```python
from build123d import *

# Parameters (mm, degrees)
F0_W      = 12
F0_H      = 10
F1_DEPTH  = 3.3
F2_SIZE   = 2
F3_R      = 3
F4_R      = 3
F5_R      = 1.75
F6_DEPTH  = 25
F7_R      = 2.5
F8_DEPTH  = 25
F9_R      = 4.5
F10_DEPTH = 25
F10_TAPER = 10


with BuildPart() as f1:
    # F0 (on Top) → F1 (new body)
    with BuildSketch(Plane.XY):
        Polygon((15, -41), (15, 41), (3, 41), (-15, 41), (-15, -41), (-3, -41), align=None)
        with Locations((9, 46)):
            Rectangle(F0_W, F0_H)
        with Locations((-9, -46)):
            Rectangle(F0_W, F0_H)
    extrude(amount=F1_DEPTH)

    # F2
    f2_edges = [f1.edges().sort_by_distance(p)[0] for p in [
        (15, 51, 1.65),
        (3, 51, 1.65),
        (-15, -51, 1.65),
        (-3, -51, 1.65),
    ]]
    chamfer(f2_edges, length=F2_SIZE)

    # F3
    f3_edges = [f1.edges().sort_by_distance(p)[0] for p in [
        (3, 41, 1.65),
    ]]
    fillet(f3_edges, radius=F3_R)

    # F4
    f4_edges = [f1.edges().sort_by_distance(p)[0] for p in [
        (-3, -41, 1.65),
    ]]
    fillet(f4_edges, radius=F4_R)

    # F5 (on face) → F6 (cut)
    with BuildSketch(Plane.XY.offset(3.3)):
        with Locations((9, 46)):
            Circle(F5_R)
        with Locations((-9, -46)):
            Circle(F5_R)
    extrude(amount=-F6_DEPTH, mode=Mode.SUBTRACT)

    # F7 (on face) → F8 (cut)
    with BuildSketch(Plane.XY.offset(3.3)):
        with Locations((0, 26)):
            Circle(F7_R)
        with Locations((0, -26)):
            Circle(F7_R)
    extrude(amount=-F8_DEPTH, mode=Mode.SUBTRACT)

    # F9 (on face) → F10 (cut)
    with BuildSketch(Plane.XY.offset(3.3)):
        with Locations((0, 26)):
            Circle(F9_R)
        with Locations((0, -26)):
            Circle(F9_R)
    extrude(amount=-F10_DEPTH, taper=F10_TAPER, mode=Mode.SUBTRACT)


solid = f1.part
```
Read the model definition and answer for the solid it produces. Units are mm, in the model's axes. A direction names the side the tool comes from. Give positions to 0.01 mm unless a question says otherwise; leave off trailing zeros. Loops run counter-clockwise (first coordinate to the right, second up) from the corner with the lowest first, then second, coordinate; pieces in that order, holes last.
Item 1: The part is cut by section B-B (y = 46). Write down the section's boundary in (x, z).
Item 2: The mould has two halves that part along Y. Classify faces 1 (the conical face through (-0.88, -29.98, 0.89)), 2 (the cylindrical face through (-2.1, -41.86, 1.67)), 3 (the flat face through (-15, -3, 2)): released by +Y, released by -Y, zero draft, split by the parting line, or undercut.
Item 3: The part is cut by section A-A (x = 9). Write down the section's boundary in (y, z).
Item 4: The part is cut by section C-C (z = 2.3). Write down the section's boundary in (x, y).
Item 5: Each of these flat-tipped pins is pushed along its axis until it touches: pin 1 Ø1 at (x, z) = (5.5, 1) entering from -Y; pin 2 Ø1.6 at (y, z) = (-47, 1) entering from +X; pin 3 Ø1 at (y, z) = (47, 2) entering from -X. Where does it stop, or does it pass through?
Item 6: For faces 4 (the flat face through (3, 46, 2)), 5 (the flat face through (7, -41, 2)), 6 (the cylindrical face through (8.62, 44.29, 1.67)), determine the directions among +Z, -Z, +X, -X, +Y, -Y from which every point of the face is accessible in a straight line to the end or side of a thin tool.
Item 7: Find the intervals of material crossed by line 1 along Y through (x, z) = (9, 2.15); line 2 along Y through (x, z) = (-3.5, 2.3); line 3 along Y through (x, z) = (-8.75, 1.2), in increasing order.
Taken from the geometry:
1. outline: (3, 0) - (7.25, 0) - (7.25, 3.3) - (3, 3.3) - close; (10.75, 0) - (15, 0) - (15, 3.3) - (10.75, 3.3) - close
2. face 1: undercut
2. face 2: released by -Y
2. face 3: zero draft
3. outline: (-41, 0) - (44.25, 0) - (44.25, 3.3) - (-41, 3.3) - close; (47.75, 0) - (51, 0) - (51, 3.3) - (47.75, 3.3) - close
4. outline: (-15, -49) - (-13, -51) - (-5, -51) - (-3, -49) - (-3, -44) arc R3 cw to (0, -41) - (15, -41) - (15, 49) - (13, 51) - (5, 51) - (3, 49) - (3, 44) arc R3 cw to (0, 41) - (-15, 41) - close; hole circle Ø3.5 at (-9, -46); hole circle Ø8.65 at (0, -26); hole circle Ø8.65 at (0, 26); hole circle Ø3.5 at (9, 46)
5. pin 1: stops at y = -41
5. pin 2: stops at x = -3
5. pin 3: stops at x = 3
6. face 4: +Z, -Z, -X, +Y
6. face 5: +Z, -Z, +X, -Y
6. face 6: +Z, -Z
7. line 1: y = -41 to 44.25, 47.75 to 51
7. line 2: y = -49.5 to -28.54, -23.46 to 23.46, 28.54 to 41
7. line 3: y = -51 to -47.73, -44.27 to 41
